Check sheet for the modelled part. Datum: model origin and axes. Units: mm. A direction names the side the tool comes from. Give positions to 0.01 mm unless a question says otherwise; leave off trailing zeros. Loops run counter-clockwise (first coordinate to the right, second up) from the corner with the lowest first, then second, coordinate; pieces in that order, holes last.
```python
from build123d import *

# Parameters (mm, degrees)
F1_DEPTH = 19.05
F2_R     = 2.6162
F3_DEPTH = 25.4
F4_R     = 2.6162
F5_DEPTH = 25.4


with BuildPart() as f1:
    # F0 (on Right) → F1 (new body)
    with BuildSketch(Plane.YZ):
        Polygon((0, -17.4625), (0, 0), (-1.5875, 0), (-1.5875, -19.05), (17.4625, -19.05), (17.4625, -17.4625), align=None)
    extrude(amount=-F1_DEPTH)

    # F2 (on face) → F3 (cut)
    with BuildSketch(Plane.XY.offset(-17.4625)):
        with Locations((-10.3378, 8.73125)):
            Circle(F2_R)
    extrude(amount=-F3_DEPTH, mode=Mode.SUBTRACT)

    # F4 (on face) → F5 (cut)
    with BuildSketch(Plane(origin=(0, 0, 0), x_dir=(-1, 0, 0), z_dir=(0, 1, 0))):
        with Locations((10.3378, -8.73125)):
            Circle(F4_R)
    extrude(amount=-F5_DEPTH, mode=Mode.SUBTRACT)


solid = f1.part
```
(1) Section check D-D on x = -13.75. Record the boundary of the cut face in (y, z), plus the area to 3 significant figures.
(2) Section check A-A on x = -8.5. Record the boundary of the cut face in (y, z), plus the area to 3 significant figures.
(3) Section check B-B on y = 10.5. Record the boundary of the cut face in (x, z), plus the area to 3 significant figures.
(4) Release check for a two-part mould opening along X. For faces 1 (the face through (-19.05, -1, -14)), 2 (the face through (-9, -1.588, -12)), 3 (the face through (-12.833, -0.783, -7.945)) record: pulls with the +X half, pulls with the -X half, needs draft (parallel to the pull), parting line crosses it, or undercut.
(5) Section check C-C on z = -8. Record the boundary of the cut face in (x, y).
(6) Access from +Z, -Z, +X, -X, +Y, -Y to the whole of each face (thin tool, end or side, straight path). Record for faces 4 (the face through (-7.842, 9.517, -18.245)), 5 (the face through (-7, 9, -17.462)).
(7) Gauge pin test, flat ends, axial feed: pin 1 Ø8.5 at (x, y) = (-10.34, 8.73) entering from +Z; pin 2 Ø1 at (x, z) = (-4, -15.5) entering from +Y. Record the tip position at first contact, or that the pin passes through.
(8) Material ranges on line 1 (Z direction, x = -12, y = 0.25); line 2 (Y direction, x = -5, z = -17.25), recorded low to high.
Computed values:
1. outline: (-1.59, -19.05) - (17.46, -19.05) - (17.46, -17.46) - (0, -17.46) - (0, 0) - (-1.59, 0) - close
1. area: 58.0 mm2
2. outline: (-1.59, -19.05) - (6.87, -19.05) - (6.87, -17.46) - (0, -17.46) - (0, -10.59) - (-1.59, -10.59) - close; (-1.59, -6.87) - (0, -6.87) - (0, 0) - (-1.59, 0) - close; (10.59, -19.05) - (17.46, -19.05) - (17.46, -17.46) - (10.59, -17.46) - close
2. area: 46.1 mm2
3. outline: (-19.05, -19.05) - (-12.27, -19.05) - (-12.27, -17.46) - (-19.05, -17.46) - close; (-8.41, -19.05) - (0, -19.05) - (0, -17.46) - (-8.41, -17.46) - close
3. area: 24.1 mm2
4. face 1: pulls with the -X half
4. face 2: needs draft
4. face 3: undercut
5. outline: (-19.05, -1.59) - (-12.85, -1.59) - (-12.85, 0) - (-19.05, 0) - close; (-7.83, -1.59) - (0, -1.59) - (0, 0) - (-7.83, 0) - close
6. face 4: +Z, -Z
6. face 5: +Z, +X, -X, +Y
7. pin 1: stops at z = -17.46
7. pin 2: stops at y = 0
8. line 1: z = -19.05 to -17.46
8. line 2: y = -1.59 to 0
